Read the model definition and answer for the solid it produces. Units are mm, in the model's axes. Face numbers are marked on the shaded views. A direction names the side the tool comes from. Give positions to 0.01 mm unless a question says otherwise; leave off trailing zeros. Write each loop counter-clockwise with the first axis right and the second up, starting at its lowest first coordinate (ties: lowest second). Pieces come first, ordered by that corner, then holes. Notation, with made-up numbers: M 57.25,79.25 L 100.25,79.25 A13 cw 100.25,87.25 Z; hole C 46,64.5 d11. An arc over 180 degrees is marked long. Use a Markdown table: item, result. Add a question column.
Item 1: Consider probe 1 along X at (y, z) = (-22, 200); probe 2 along Y at (x, z) = (-54.5, 123); probe 3 along Z at (x, y) = (36, -27.5). Determine where each line is inside the solid, lowest interval first. Write a range as [from, to].
Item 2: A cutting plane is placed at B-B on y = -18.5. Determine the outline of the cut face in (x, z), then the cut area to 3 significant figures.
Item 3: For the marked faces 1 and 2, determine the directions among +Z, -Z, +X, -X, +Y, -Y from which every point of the face is accessible in a straight line to the end or side of a thin tool.
Item 4: A cutting plane is placed at C-C on y = -83. Determine the outline of the cut face in (x, z).
Item 5: A cutting plane is placed at D-D on z = 106.5. Determine the outline of the cut face in (x, y).
Item 6: A cutting plane is placed at A-A on z = 76. Determine the outline of the cut face in (x, y), then the cut area to 3 significant figures.
Item 7: Given P1, Ø3, axis at x = 52, z = 263.5, coming from the -Y side; P2, Ø9.5, axis at x = 75.91, z = 200, coming from the -Y side; P3, Ø1, axis at y = -11.5, z = 257.5, coming from the +X side; P4, Ø1.5, axis at y = -25, z = 234.5, coming from the -X side, each flat-ended and moving along its own axis, determine where each tip first touches the part or whether it passes through.
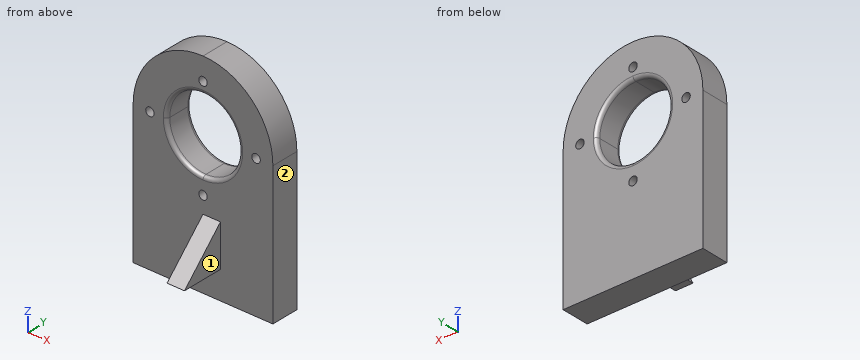
from build123d import *

# Parameters (mm, degrees)
F1_DEPTH = 40
F2_D     = 12.1
F3_R     = 5
F4_R     = 5
F6_DEPTH = 25


with BuildPart() as f1:
    # F0 (on Front) → F1 (new body)
    with BuildSketch(Plane.XZ):
        with BuildLine():
            Line((-100, 0), (0, 0))
            Line((0, 0), (0, 100))
            ThreePointArc((0, 100), (-70.7106781187, 129.2893218813), (-100, 200))
            Line((-100, 200), (-100, 0))
        make_face()
        with BuildLine():
            Line((0, 100), (0, 0))
            Line((0, 0), (100, 0))
            Line((100, 0), (100, 200))
            ThreePointArc((100, 200), (70.7106781187, 129.2893218813), (0, 100))
        make_face()
        with BuildLine():
            ThreePointArc((-100, 200), (-70.7106781187, 129.2893218813), (0, 100))
            Line((0, 100), (0, 148.1840150042))
            ThreePointArc((0, 148.1840150042), (-36.6394343644, 163.3605656356), (-51.8159849958, 200))
            Line((-51.8159849958, 200), (-100, 200))
        make_face()
        with BuildLine():
            Line((0, 148.1840150042), (0, 100))
            ThreePointArc((0, 100), (70.7106781187, 129.2893218813), (100, 200))
            Line((100, 200), (51.8159849958, 200))
            ThreePointArc((51.8159849958, 200), (36.6394343644, 163.3605656356), (0, 148.1840150042))
        make_face()
        with BuildLine():
            ThreePointArc((0, 300), (-70.7106781187, 270.7106781187), (-100, 200))
            Line((-100, 200), (-51.8159849958, 200))
            ThreePointArc((-51.8159849958, 200), (-36.6394343644, 236.6394343644), (0, 251.8159849958))
            Line((0, 251.8159849958), (0, 300))
        make_face()
        with BuildLine():
            Line((51.8159849958, 200), (100, 200))
            ThreePointArc((100, 200), (70.7106781187, 270.7106781187), (0, 300))
            Line((0, 300), (0, 251.8159849958))
            ThreePointArc((0, 251.8159849958), (36.6394343644, 236.6394343644), (51.8159849958, 200))
        make_face()
    extrude(amount=F1_DEPTH)

    # F2 (through all)
    with Locations(Plane(origin=(0, 0, 0), x_dir=(1, 0, 0), z_dir=(0, 1, 0))):
        with Locations((-75.9079924979, -200), (0, -267.9978298545), (75.9079924979, -200), (0, -123.9978298545)):
            Hole(F2_D / 2)

    # F3
    f3_edges = [f1.edges().sort_by_distance(p)[0] for p in [
        (0, -40, 148.184015),
    ]]
    fillet(f3_edges, radius=F3_R)

    # F4
    f4_edges = [f1.edges().sort_by_distance(p)[0] for p in [
        (0, 0, 148.184015),
    ]]
    fillet(f4_edges, radius=F4_R)

    # F5 (on Right) → F6 (join)
    with BuildSketch(Plane.YZ):
        Polygon((-100, 40), (-40, 40), (-40, 100), align=None)
    extrude(amount=F6_DEPTH)


solid = f1.part
Filled in:
| question | item | result |
|---|---|---|
| 1 | probe 1 | [-100, -81.96], [-69.86, -51.82], [51.82, 69.86], [81.96, 100] |
| 1 | probe 2 | [-40, 0] |
| 1 | probe 3 | [0, 162.73], [237.27, 293.3] |
| 2 | outline | M -100,0 L 100,0 L 100,200 A100 ccw -100,200 Z; hole C -75.91,200 d12.1; hole C 0,200 d103.63; hole C 0,124 d12.1; hole C 0,268 d12.1; hole C 75.91,200 d12.1 |
| 2 | area | 46,800 mm² |
| 3 | face 1 | +Z, -Z, +X, -Y |
| 3 | face 2 | +Z, -Z, +X, +Y, -Y |
| 4 | outline | M 0,40 L 25,40 L 25,57 L 0,57 Z |
| 5 | outline | M -100,-40 L 100,-40 L 100,0 L -100,0 Z |
| 6 | outline | M -100,-40 L 0,-40 L 0,-64 L 25,-64 L 25,-40 L 100,-40 L 100,0 L -100,0 Z |
| 6 | area | 8,600 mm² |
| 7 | P1 | y = -40 |
| 7 | P2 | through |
| 7 | P3 | x = 82.16 |
| 7 | P4 | x = -94.13 |
